from build123d import *

# Parameters (mm, degrees)
ESQUISSE1_R             = 25
ESQUISSE1_R_2           = 1.7
BOSS_EXTRU_1_DEPTH      = 9
ESQUISSE6_R             = 11
ENL_V_MAT_EXTRU_2_DEPTH = 6
CONG_2_R                = 0.5
ESQUISSE15_W            = 7.963879273
ESQUISSE15_H            = 27.450042448
ENL_V_MAT_EXTRU_4_DEPTH = 37.482872694
ESQUISSE16_W            = 21.21339198
ESQUISSE16_H            = 6
ENL_V_MAT_EXTRU_5_DEPTH = 6


with BuildPart() as part:
    # Esquisse1 → Boss.-Extru.1 (new body)
    with BuildSketch(Plane.XY):
        Circle(ESQUISSE1_R)
        with Locations((-13.435028843, 13.435028843)):
            Circle(ESQUISSE1_R_2, mode=Mode.SUBTRACT)
        with Locations((13.435028843, 13.435028843)):
            Circle(ESQUISSE1_R_2, mode=Mode.SUBTRACT)
        with Locations((13.435028843, -13.435028843)):
            Circle(ESQUISSE1_R_2, mode=Mode.SUBTRACT)
        with Locations((-13.435028843, -13.435028843)):
            Circle(ESQUISSE1_R_2, mode=Mode.SUBTRACT)
    extrude(amount=BOSS_EXTRU_1_DEPTH)

    # Esquisse6 → Enlèv. mat.-Extru.2 (cut)
    with BuildSketch(Plane(origin=(0, 0, 0), x_dir=(-1, 0, 0), z_dir=(0, 0, -1))):
        Circle(ESQUISSE6_R)
    extrude(amount=-ENL_V_MAT_EXTRU_2_DEPTH, mode=Mode.SUBTRACT)

    # Congé2
    cong_2_edges = [part.edges().sort_by_distance(p)[0] for p in [
        (11, 0, 6),
    ]]
    fillet(cong_2_edges, radius=CONG_2_R)

    # Esquisse15 → Enlèv. mat.-Extru.4 (cut, through all)
    with BuildSketch(Plane(origin=(0, 0, 0), x_dir=(-1, 0, 0), z_dir=(0, 0, -1))):
        with Locations((-25.065108278, -0.289992381)):
            Rectangle(ESQUISSE15_W, ESQUISSE15_H)
    extrude(amount=-ENL_V_MAT_EXTRU_4_DEPTH, mode=Mode.SUBTRACT)

    # Esquisse16 → Enlèv. mat.-Extru.5 (cut)
    with BuildSketch(Plane(origin=(0, 0, 0), x_dir=(-1, 0, 0), z_dir=(0, 0, -1))):
        with Locations((17.506358801, 0)):
            Rectangle(ESQUISSE16_W, ESQUISSE16_H)
    extrude(amount=-ENL_V_MAT_EXTRU_5_DEPTH, mode=Mode.SUBTRACT)


solid = part.part
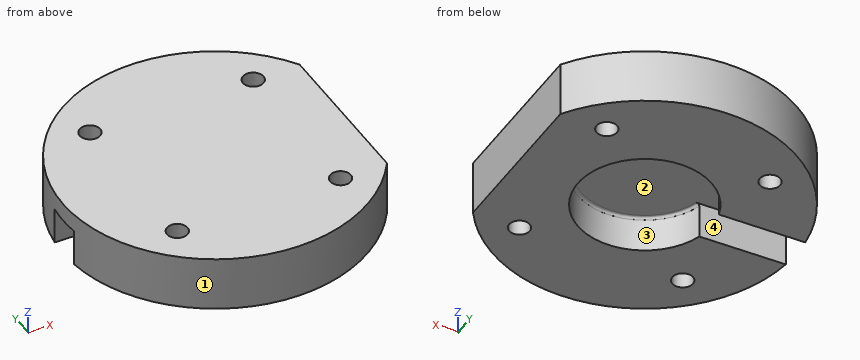
Build history of the part. All positions in model axes, mm. Face numbers are marked on the shaded views. Round coordinates to 2 decimals unless told otherwise and drop trailing zeros. Write each loop counter-clockwise with the first axis right and the second up, starting at its lowest first coordinate (ties: lowest second). Pieces come first, ordered by that corner, then holes. Notation, with made-up numbers: (17, 88.5) - (22, 88.5) arc R17 cw to (22, 119.5) - close; hole circle Ø8 at (40.25, 22.5). An arc over 180 degrees is marked (long way). One line per question, with ' | ' between items.
1. Drop flat-ended pins along their axis: pin 1 Ø2 at (x, y) = (-13.44, -13.44) entering from +Z; pin 2 Ø5.5 at (x, y) = (13.44, -13.44) entering from +Z; pin 3 Ø3 at (x, z) = (-16, 1.5) entering from -Y; pin 4 Ø5 at (x, z) = (14, 2.5) entering from +Y. Give the stop position or say it passes through.
Results are:
pin 1: through | pin 2: z = 9 | pin 3: y = -20.37 | pin 4: y = 22.2
2. Band-saw the part on C-C, the plane x = 0. Write the cut outline in (y, z), and give its area (3 significant figures).
Results are:
outline: (-25, 0) - (-11, 0) - (-11, 5.5) arc R0.5 cw to (-10.5, 6) - (10.5, 6) arc R0.5 cw to (11, 5.5) - (11, 0) - (25, 0) - (25, 9) - (-25, 9) - close | area: 318 mm^2
3. Band-saw the part on B-B, the plane z = 2.25. Write the cut outline in (x, y).
Results are:
outline: (-24.82, -3) arc R25 ccw to (21.08, -13.44) - (21.08, 13.44) arc R25 ccw to (-24.82, 3) - (-10.58, 3) arc R11 cw (long way) to (-10.58, -3) - close; hole circle Ø3.4 at (-13.44, -13.44); hole circle Ø3.4 at (-13.44, 13.44); hole circle Ø3.4 at (13.44, -13.44); hole circle Ø3.4 at (13.44, 13.44)
4. Band-saw the part on D-D, the plane x = -13. Write the cut outline in (y, z).
Results are:
outline: (-21.35, 0) - (-15.08, 0) - (-15.08, 9) - (-21.35, 9) - close; (-11.79, 0) - (-3, 0) - (-3, 6) - (3, 6) - (3, 0) - (11.79, 0) - (11.79, 9) - (-11.79, 9) - close; (15.08, 0) - (21.35, 0) - (21.35, 9) - (15.08, 9) - close
5. Mould opens along X. For the marked faces 1, 2, 3 and 4 say: released by +X, released by -X, zero draft, split by the parting line, or undercut.
Results are:
face 1: split by the parting line | face 2: undercut | face 3: undercut | face 4: zero draft
6. Drill centre lines: line 1 along Y through (x, z) = (0, 3.25); line 2 along X through (y, z) = (-12, 6.5); line 3 along Y through (x, z) = (-14.5, 4). Where is each one in solid material? Low to high. Write a range as from..to.
Results are:
line 1: -25..-11, 11..25 | line 2: -21.93..-14.35, -12.52..12.52, 14.35..21.08 | line 3: -20.37..-14.76, -12.11..-3, 3..12.11, 14.76..20.37
7. Band-saw the part on A-A, the plane y = 0. Write the cut outline in (x, z).
Results are:
outline: (-25, 6) - (10.5, 6) arc R0.5 cw to (11, 5.5) - (11, 0) - (21.08, 0) - (21.08, 9) - (-25, 9) - close
